```python
from build123d import *

# Parameters (mm, degrees)
BOSS_EXTRUDE1_DEPTH        = 7
SKETCH5_R                  = 45
CUT_EXTRUDE1_DEPTH         = 20
SKETCH6_R                  = 44
CUT_EXTRUDE3_DEPTH         = 7
SKETCH8_R                  = 39.5
CUT_EXTRUDE4_DEPTH         = 7
F_8_8_8_8_DIAMETER_HOLE1_D = 8.8
CHAMFER1_SIZE              = 1
FILLET1_R                  = 1
FILLET3_R                  = 2
FILLET4_R                  = 0.8
FILLET5_R                  = 3
BOSS_EXTRUDE2_DEPTH        = 1


with BuildPart() as part:
    # Sketch1 → Boss-Extrude1 (new body)
    with BuildSketch(Plane(origin=(0, 0, 0), x_dir=(1, 0, 0), z_dir=(0, 1, 0))):
        with BuildLine():
            Line((-40.001844064, 56.369319939), (40.001844064, 56.369319939))
            ThreePointArc((40.001844064, 56.369319939), (44.757455682, 55.010272637), (48.076822603, 51.343577304))
            Line((48.076822603, 51.343577304), (70.011643797, 6.775952684))
            ThreePointArc((70.011643797, 6.775952684), (70.931678065, 2.502121267), (69.729322621, -1.701025105))
            Line((69.729322621, -1.701025105), (36.296218849, -59.56220628))
            ThreePointArc((36.296218849, -59.56220628), (30.85289019, -63.747446182), (24.042134471, -62.875857711))
            ThreePointArc((24.042134471, -62.875857711), (0, -56.497417156), (-24.042134471, -62.875857711))
            ThreePointArc((-24.042134471, -62.875857711), (-30.85289019, -63.747446182), (-36.296218849, -59.56220628))
            Line((-36.296218849, -59.56220628), (-69.729322621, -1.701025105))
            ThreePointArc((-69.729322621, -1.701025105), (-70.931678065, 2.502121267), (-70.011643797, 6.775952684))
            Line((-70.011643797, 6.775952684), (-48.076822603, 51.343577304))
            ThreePointArc((-48.076822603, 51.343577304), (-44.757455682, 55.010272637), (-40.001844064, 56.369319939))
        make_face()
    extrude(amount=BOSS_EXTRUDE1_DEPTH)

    # Sketch4 → Revolve2 (revolve)
    with BuildSketch(Plane(origin=(0, 0, 0), x_dir=(0, 0, -1), z_dir=(1, 0, 0))):
        Polygon((0, 0), (0, 34), (53, 34), (53, 23.333628962), (54.924671579, 20), (54.924671579, 0), align=None)
    revolve(axis=Axis((0, 0, 0), (0, 1, 0)))

    # Sketch5 → Cut-Extrude1 (cut)
    with BuildSketch(Plane(origin=(0, 34, 0), x_dir=(1, 0, 0), z_dir=(0, 1, 0))):
        with Locations(Location((0, 0, 0), (0, 0, 270))):
            Circle(SKETCH5_R)
    extrude(amount=-CUT_EXTRUDE1_DEPTH, mode=Mode.SUBTRACT)

    # Sketch6 → Cut-Extrude3 (cut)
    with BuildSketch(Plane(origin=(0, 14, 0), x_dir=(1, 0, 0), z_dir=(0, 1, 0))):
        with Locations(Location((0, 0, 0), (0, 0, 270))):
            Circle(SKETCH6_R)
    extrude(amount=-CUT_EXTRUDE3_DEPTH, mode=Mode.SUBTRACT)

    # Sketch8 → Cut-Extrude4 (cut)
    with BuildSketch(Plane(origin=(0, 7, 0), x_dir=(1, 0, 0), z_dir=(0, 1, 0))):
        with Locations(Location((0, 0, 0), (0, 0, 270))):
            Circle(SKETCH8_R)
    extrude(amount=-CUT_EXTRUDE4_DEPTH, mode=Mode.SUBTRACT)

    # Ø8.8 (8.8) Diameter Hole1 (through all)
    with Locations(Plane(origin=(0, 7, 0), x_dir=(1, 0, 0), z_dir=(0, 1, 0))):
        with Locations((-62, 0), (62, 0), (28.503561486, -55.059485855), (-28.503561486, -55.059485855), (-40.001844064, 47.369319939), (40.001844064, 47.369319939)):
            Hole(F_8_8_8_8_DIAMETER_HOLE1_D / 2)

    # Chamfer1
    chamfer1_edges = [part.edges().sort_by_distance(p)[0] for p in [
        (0, 34, -45),
    ]]
    chamfer(chamfer1_edges, length=CHAMFER1_SIZE)

    # Fillet1
    fillet1_edges = [part.edges().sort_by_distance(p)[0] for p in [
        (0, 34, 53),
    ]]
    fillet(fillet1_edges, radius=FILLET1_R)

    # Fillet3
    fillet3_edges = [part.edges().sort_by_distance(p)[0] for p in [
        (0, 0, -39.5),
    ]]
    fillet(fillet3_edges, radius=FILLET3_R)

    # Fillet4
    fillet4_edges = [part.edges().sort_by_distance(p)[0] for p in [
        (0, 7, 54.924671579),
    ]]
    fillet(fillet4_edges, radius=FILLET4_R)

    # Fillet5
    fillet5_edges = [part.edges().sort_by_distance(p)[0] for p in [
        (0, 7, -39.5),
    ]]
    fillet(fillet5_edges, radius=FILLET5_R)

    # Sketch14 → Boss-Extrude2 (add)
    # profile 1 of 6: a face of its own
    with BuildSketch(Plane.XZ):
        Polygon((-49.543668777, -15.701397917), (-52.160255315, -18.505885097), (-52.299778552, -18.160232052), (-51.443708841, -17.225636699), (-52.004606277, -15.836013302), (-53.268728873, -15.76099327), (-53.413861085, -15.401317789), (-49.575920379, -15.622171154), align=None)
        Polygon((-50.243388328, -15.937675962), (-51.635115091, -15.855644712), (-51.190603873, -16.957808174), align=None, mode=Mode.SUBTRACT)
    # profile 2 of 6: a face of its own
    with BuildSketch(Plane.XZ):
        with BuildLine():
            Line((-51.952551008, -19.013684924), (-48.729494117, -17.711701751))
            Line((-48.729494117, -17.711701751), (-48.459562226, -18.380571943))
            add(Edge.make_bspline(
                [(-48.459562226, -18.380571943), (-48.436319484, -18.438869332), (-48.391527252, -18.551217098), (-48.332197088, -18.715837983), (-48.279869356, -18.868901378), (-48.236746224, -19.011472904), (-48.203016387, -19.143227311), (-48.177589166, -19.263893851), (-48.159744735, -19.37360661), (-48.15480571, -19.443421596), (-48.15247088, -19.476425309)],
                knots=[0, 0, 0, 0, 1.318128298, 2.540229846, 3.674976834, 4.715486728, 5.667951583, 6.530565877, 7.305352836, 8, 8, 8, 8], degree=3))
            add(Edge.make_bspline(
                [(-48.15247088, -19.476425309), (-48.151224452, -19.520606977), (-48.148768191, -19.607673125), (-48.158604762, -19.736863905), (-48.177290489, -19.862545907), (-48.20614634, -19.985268532), (-48.245237679, -20.104583309), (-48.295722785, -20.220129151), (-48.355312524, -20.33252403), (-48.42475478, -20.441047803), (-48.503132327, -20.544811018), (-48.590432451, -20.642263928), (-48.685411525, -20.734142298), (-48.78945408, -20.81872348), (-48.901448884, -20.897257962), (-49.020847396, -20.970773883), (-49.149325985, -21.036528429), (-49.239194617, -21.074600395), (-49.284782579, -21.093913289)],
                knots=[0, 0, 0, 0, 1.002436367, 1.975440866, 2.935524168, 3.883623185, 4.832893364, 5.780695656, 6.741584304, 7.7170141, 8.701371253, 9.689279608, 10.683262391, 11.697138007, 12.728616468, 13.785564042, 14.876675657, 16, 16, 16, 16], degree=3))
            add(Edge.make_bspline(
                [(-49.284782579, -21.093913289), (-49.324815131, -21.109331789), (-49.403899502, -21.139791059), (-49.523778301, -21.176870412), (-49.642767374, -21.205680865), (-49.760487205, -21.227015821), (-49.877418114, -21.239561485), (-49.993338957, -21.244479251), (-50.108405872, -21.242004451), (-50.221706432, -21.23038608), (-50.332343223, -21.212575154), (-50.438930962, -21.186883076), (-50.541509718, -21.156494998), (-50.639349049, -21.118977336), (-50.732988708, -21.075859162), (-50.821324957, -21.024799667), (-50.905855004, -20.968661326), (-50.986930076, -20.905886064), (-51.063640011, -20.833392499), (-51.138502103, -20.751644166), (-51.210394991, -20.658684386), (-51.280555312, -20.555374378), (-51.34830296, -20.441286466), (-51.415042693, -20.317333909), (-51.478782823, -20.182378875), (-51.518013915, -20.087973122), (-51.538188027, -20.03942611)],
                knots=[0, 0, 0, 0, 1.089389366, 2.15209041, 3.184381895, 4.197412583, 5.188571916, 6.168900145, 7.142700834, 8.10901874, 9.05952745, 9.986767119, 10.891931066, 11.774986155, 12.646048741, 13.5074912, 14.363599599, 15.222112427, 16.108254607, 17.041026014, 18.034901271, 19.09026574, 20.211109633, 21.403560202, 22.66481235, 24, 24, 24, 24], degree=3))
            Line((-51.538188027, -20.03942611), (-51.952551008, -19.013684924))
        make_face()
        with BuildLine():
            Line((-51.52346447, -19.200183321), (-51.373424406, -19.572478994))
            add(Edge.make_bspline(
                [(-51.373424406, -19.572478994), (-51.351687068, -19.625861431), (-51.309857596, -19.728586024), (-51.245995509, -19.874794681), (-51.185358504, -20.007631691), (-51.126477819, -20.126080253), (-51.070447188, -20.230898537), (-51.017349895, -20.321989806), (-50.967611746, -20.400034109), (-50.93205766, -20.444920434), (-50.915591873, -20.465708161)],
                knots=[0, 0, 0, 0, 1.373973852, 2.643957675, 3.803132799, 4.854571426, 5.796777433, 6.63573208, 7.368181077, 8, 8, 8, 8], degree=3))
            add(Edge.make_bspline(
                [(-50.915591873, -20.465708161), (-50.893067449, -20.491076278), (-50.848579246, -20.541181086), (-50.775849059, -20.609380616), (-50.699586198, -20.670612056), (-50.618798321, -20.723974157), (-50.534992901, -20.77166449), (-50.445875983, -20.809543603), (-50.353897644, -20.842519476), (-50.257820072, -20.866646744), (-50.159162967, -20.883695793), (-50.058287851, -20.891826428), (-49.955849846, -20.892723152), (-49.851758396, -20.884830378), (-49.746062391, -20.868565655), (-49.638926588, -20.843633305), (-49.529789733, -20.811760922), (-49.458011128, -20.784076534), (-49.421501329, -20.76999502)],
                knots=[0, 0, 0, 0, 0.99342231, 1.962117752, 2.916971191, 3.85503458, 4.796016756, 5.737297783, 6.687895217, 7.65600979, 8.6352695, 9.617778921, 10.617410475, 11.633506781, 12.672504164, 13.747098093, 14.854073601, 16, 16, 16, 16], degree=3))
            add(Edge.make_bspline(
                [(-49.421501329, -20.76999502), (-49.383641237, -20.753905877), (-49.308922936, -20.722153354), (-49.202690032, -20.666608393), (-49.103129906, -20.606294537), (-49.011211685, -20.540174357), (-48.925893295, -20.469227129), (-48.847683766, -20.392838655), (-48.777686199, -20.31009173), (-48.713598524, -20.223688802), (-48.658266213, -20.132259656), (-48.61120855, -20.037798765), (-48.573086878, -19.940158697), (-48.543431996, -19.83982122), (-48.523320599, -19.736256133), (-48.511213396, -19.629838407), (-48.508367186, -19.52050369), (-48.513207587, -19.446958665), (-48.51565197, -19.409818738)],
                knots=[0, 0, 0, 0, 1.120915847, 2.212169129, 3.264268614, 4.2913861, 5.295427879, 6.286451793, 7.266916285, 8.246718328, 9.215775873, 10.175851217, 11.119857042, 12.069285214, 13.023764875, 13.991753987, 14.985844258, 16, 16, 16, 16], degree=3))
            add(Edge.make_bspline(
                [(-48.51565197, -19.409818738), (-48.518947599, -19.379603205), (-48.525987362, -19.31506008), (-48.546867029, -19.213757546), (-48.573321082, -19.100883292), (-48.608745038, -18.97730872), (-48.651786281, -18.842498512), (-48.70224613, -18.6965188), (-48.761515015, -18.539743047), (-48.804141475, -18.431699133), (-48.826248925, -18.375664091)],
                knots=[0, 0, 0, 0, 0.673256086, 1.438136185, 2.289883846, 3.242504658, 4.285922505, 5.425944978, 6.665012424, 8, 8, 8, 8], degree=3))
            Line((-48.826248925, -18.375664091), (-48.91809588, -18.147799507))
            Line((-48.91809588, -18.147799507), (-51.52346447, -19.200183321))
        make_face(mode=Mode.SUBTRACT)
    # profile 3 of 6: a face of its own
    with BuildSketch(Plane.XZ):
        Polygon((-47.401397182, -20.99384052), (-47.27168965, -21.315655424), (-50.494746541, -22.617638597), (-50.624454073, -22.295823693), align=None)
    # profile 4 of 6: a face of its own
    with BuildSketch(Plane.XZ):
        Polygon((-47.421678037, -21.844918449), (-47.108276595, -21.718015405), (-46.394534607, -23.486244571), (-46.70793605, -23.613147616), (-46.998200473, -22.894497776), (-49.907855922, -24.069577905), (-50.040367941, -23.740751783), (-47.130712492, -22.565671655), align=None)
    # profile 5 of 6: a face of its own
    with BuildSketch(Plane.XZ):
        Polygon((-46.307496458, -23.697355073), (-46.157456394, -24.069650746), (-47.152348221, -25.429827028), (-45.497700785, -25.70396565), (-45.346959599, -26.076962445), (-47.441911522, -25.735516131), (-48.982276105, -26.357411163), (-49.110581394, -26.039802989), (-47.57021681, -25.417907957), align=None)
    # profile 6 of 6: a face of its own
    with BuildSketch(Plane.XZ):
        Polygon((-44.595920352, -27.930738364), (-47.21250689, -30.735225544), (-47.352030127, -30.389572499), (-46.495960416, -29.454977146), (-47.056857852, -28.065353749), (-48.320980448, -27.990333717), (-48.466112659, -27.630658236), (-44.628171954, -27.851511601), align=None)
        Polygon((-45.295639903, -28.167016409), (-46.687366666, -28.084985159), (-46.242855448, -29.187148621), align=None, mode=Mode.SUBTRACT)
    extrude(amount=BOSS_EXTRUDE2_DEPTH)


solid = part.part
```
Design review of the part built by this model. Coordinates are the model's own, in mm. A direction names the side the tool comes from. Coordinates: 2 decimals unless noted, no trailing zeros. Order: outer loops, then holes, each group sorted by start corner. A loop starts at its lowest first (then second) coordinate and runs counter-clockwise, first axis right, second up.
1) Clearance check with flat-ended pins moving along their axes: pin 1 (1.5 mm diameter, centred on x = -31, y = 20, fed in from +Z); pin 2 (4 mm diameter, centred on x = 33.5, y = 3, fed in from +Z); pin 3 (1 mm diameter, centred on x = 25, y = 20, fed in from -Z). State where each tip first meets the part, or that it passes through.
2) Wall thickness on line 1 along Z through (x, y) = (-14, 28.5); line 2 along Y through (x, z) = (-31.5, 28.5); line 3 along Z through (x, y) = (-20, 19): over which ranges is each line inside the solid? List them lowest first.
3) Mouldability with a two-part tool opening along Z and no side actions: class faces 1 (the flat face through (-52.8, 3.5, 31)), 2 (the flat face through (-51.6, -1, -16.4)), 3 (the cylindrical face through (29.1, 3.5, 50.7)) as +Z half, -Z half, draft (parallel to the pull), parting line (faces both ways), or undercut.
4) Take a section at C-C, the plane x = -62. Give the boundary of the cut face in (y, z).
5) Take a section at B-B, the plane y = 16.5. Give the boundary of the cut face in (x, z), and give its area (3 significant figures).
6) Take a section at D-D, the plane z = 0. State how many separate pieces and enclosed holes the cut face has, and give its area (3 significant figures).
7) For faces 4 (the cylindrical face through (33.4, 13.8, 43.6)), 5 (the cylindrical face through (44.698, 3.451, -55.047)), list the 3-axis set-ups (+Z, -Z, +X, -X, +Y, -Y) from which the entire face can be reached by the end or side of a thin tool; tool diameter is ignored.
Returned:
1. pin 1: stops at z = 45.84
1. pin 2: stops at z = 63.55
1. pin 3: stops at z = -49.16
2. line 1: z = -51.12 to -42.77, 42.77 to 51.12
2. line 2: y = 0 to 7
2. line 3: z = -51.15 to -40.31, 40.31 to 51.15
3. face 1: +Z half
3. face 2: draft
3. face 3: undercut
4. outline: (0, -23.05) - (7, -23.05) - (7, -4.4) - (0, -4.4) - close; (0, 4.4) - (7, 4.4) - (7, 15.08) - (0, 15.08) - close
5. outline: circle Ø109.85 at (0, 0); hole circle Ø90 at (0, 0)
5. area: 3,120 mm2
6. separate pieces: 4
6. enclosed holes: 0
6. area: 806 mm2
7. face 4: +Y
7. face 5: -Z, +X, +Y, -Y
